Model file for the job. Use its own axes, mm. A direction names the side the tool comes from. Coordinates: 2 decimals unless noted, no trailing zeros. Write each loop counter-clockwise with the first axis right and the second up, starting at its lowest first coordinate (ties: lowest second). Pieces come first, ordered by that corner, then holes. Notation, with made-up numbers: M 12.25,22 L 51.25,22 A7 cw 51.25,31 Z; hole C 82.5,66 d8. An arc over 180 degrees is marked long. One line per question, with ' | ' between items. Start each with the question number.
(1) Tool access for faces 4 (the face through (0, -18.115, 10)), 5 (the face through (-1, 23, 20)), 6 (the face through (7, -8.115, 10)), 7 (the face through (-5, -25, 3)), 8 (the face through (0.22, 43.255, 9.86)): list every direction of +Z, -Z, +X, -X, +Y, -Y with a clear straight run to the whole face (end or side of a thin tool).
(2) Cut at D-D (y = 28.5). Write the cut outline in (x, z), plus the area to 3 significant figures.
(3) Flat gauge pins, fed straight in: pin 1 Ø6 at (y, z) = (20.5, 6.5) entering from +X; pin 2 Ø3 at (x, z) = (-26.5, 14) entering from -Y; pin 3 Ø18 at (x, y) = (-25, 33.88) entering from -Z; pin 4 Ø5.5 at (x, z) = (-7.5, 8) entering from -Y. Where does each tip first touch, or does it go through?
(4) Cut at B-B (x = 25). Write the cut outline in (y, z).
(5) Cut at A-A (y = -37.5). Write the cut outline in (x, z).
(6) Two-plate mould, pull along Y, no slides. Class faces 1 (the face through (-1, 23, 0)), 2 (the face through (15.462, 30.881, 9.86)), 3 (the face through (0, -53.115, 17)): +Y half, -Y half, draft (parallel to the pull), parting line (faces both ways), or undercut.
(7) Wall check: probe 1 along X at (y, z) = (26, 18); probe 2 along X at (y, z) = (37.5, 8.75); probe 3 along Y at (x, z) = (-0.5, 14.25). Give the ranges that are in metal, low to high.
(8) Cut at C-C (z = 7). Write the cut outline in (x, y).
from build123d import *

# Parameters (mm, degrees)
IZIM1_R                     = 10
Y_KSEKLIK_EKSTR_ZYON1_DEPTH = 20
IZIM3_W                     = 10
IZIM3_H                     = 35
KES_EKSTR_ZYON1_DEPTH       = 10


with BuildPart() as part:
    # Çizim1 → Yükseklik-Ekstrüzyon1 (new body)
    with BuildSketch(Plane.XY):
        with BuildLine():
            Line((-10, -8.115065243), (-5, -8.115065243))
            Line((-5, -8.115065243), (-5, -53.115065243))
            Line((-5, -53.115065243), (5, -53.115065243))
            Line((5, -53.115065243), (5, -8.115065243))
            Line((5, -8.115065243), (10, -8.115065243))
            ThreePointArc((10, -8.115065243), (15.132819854, 7.763816786), (29.113715132, 16.875309605))
            ThreePointArc((29.113715132, 16.875309605), (40.884337762, 41.229171535), (14.705882353, 48.037006756))
            ThreePointArc((14.705882353, 48.037006756), (0, 43.254252469), (-14.705882353, 48.037006756))
            ThreePointArc((-14.705882353, 48.037006756), (-40.884337762, 41.229171535), (-29.113715132, 16.875309605))
            ThreePointArc((-29.113715132, 16.875309605), (-15.132819854, 7.763816786), (-10, -8.115065243))
        make_face()
        with Locations((-25, 33.884934757)):
            Circle(IZIM1_R, mode=Mode.SUBTRACT)
        with Locations(Location((25, 33.884934757, 0), (0, 0, 180))):
            Circle(IZIM1_R, mode=Mode.SUBTRACT)
    extrude(amount=Y_KSEKLIK_EKSTR_ZYON1_DEPTH)

    # Çizim3 → Kes-Ekstrüzyon1 (cut)
    with BuildSketch(Plane(origin=(5, 0, 0), x_dir=(0, 0, -1), z_dir=(1, 0, 0))):
        with Locations((-10, -35.615065243)):
            Rectangle(IZIM3_W, IZIM3_H)
    extrude(amount=-KES_EKSTR_ZYON1_DEPTH, mode=Mode.SUBTRACT)


solid = part.part
Filled in:
1) face 4: +X, -X, -Y | face 5: +Z, +X, -X, +Y, -Y | face 6: +Z, -Z, +X, -Y | face 7: +Z, -Z, -X, -Y | face 8: +Z, -Z, +Y
2) outline: M -41.65,0 L -33.43,0 L -33.43,20 L -41.65,20 Z; M -16.57,0 L 16.57,0 L 16.57,20 L -16.57,20 Z; M 33.43,0 L 41.65,0 L 41.65,20 L 33.43,20 Z | area: 992 mm²
3) pin 1: x = 39.09 | pin 2: y = 15.49 | pin 3: through | pin 4: y = -18.12
4) outline: M 15.49,0 L 23.88,0 L 23.88,20 L 15.49,20 Z; M 43.88,0 L 51.38,0 L 51.38,20 L 43.88,20 Z
5) outline: M -5,0 L 5,0 L 5,5 L -5,5 Z; M -5,15 L 5,15 L 5,20 L -5,20 Z
6) face 1: draft | face 2: undercut | face 3: -Y half
7) probe 1: -40.62 to -31.15, -18.85 to 18.85, 31.15 to 40.62 | probe 2: -42.12 to -34.32, -15.68 to 15.68, 34.32 to 42.12 | probe 3: -18.12 to 43.26
8) outline: M -29.11,16.88 A25 cw -10,-8.12 L -5,-8.12 L -5,-18.12 L 5,-18.12 L 5,-8.12 L 10,-8.12 A25 cw 29.11,16.88 A17.5 ccw long 14.71,48.04 A25 cw -14.71,48.04 A17.5 ccw long Z; hole C -25,33.88 d20; hole C 25,33.88 d20
